Design review of the part built by this model. Coordinates are the model's own, in mm. A direction names the side the tool comes from. Coordinates: 2 decimals unless noted, no trailing zeros. Loops run counter-clockwise (first coordinate to the right, second up) from the corner with the lowest first, then second, coordinate; pieces in that order, holes last. Notation, with made-up numbers: (8, 44) - (52, 44) arc R4 cw to (52, 51) - close; hole circle Ø6 at (35, 86). An arc over 180 degrees is marked (long way). Use one line per item in the form item = value. Start each with the question number.
(1) Add section D-D (z = 11). State the section outline as (x, y) points.
(2) The part is to be moulded in two halves that separate along Y. For faces 5 (the face through (55, -3, 5)), 6 (the face through (-1, 12.5, 5)), 7 (the face through (0, 9, 10)), say which applies: pulls with the +Y half, pulls with the -Y half, needs draft (parallel to the pull), parting line crosses it, or undercut.
(3) Tool access review of faces 1 (the face through (-1, -10.5, 11)), 2 (the face through (57, -0.2, 4.6)), 3 (the face through (1, 0, 4)), 4 (the face through (0, 1, 7)): name each direction out of +Z, -Z, +X, -X, +Y, -Y from which nothing blocks a thin tool from reaching the whole face with its end or side.
(4) Add section B-B (y = 2). State the section outline as (x, z) points, plus the area to 3 significant figures.
(5) Clearance check with flat-ended pins moving along their axes: pin 1 Ø0.9 at (x, y) = (-55.5, -2.5) entering from +Z; pin 2 Ø0.6 at (x, z) = (2, 10.5) entering from +Y; pin 3 Ø1.5 at (x, y) = (6.5, -9.5) entering from +Z. State where each tip first meets the part, or that it passes through.
(6) For L1, parallel to X at y = 9, z = 9.25; L2, parallel to Y at x = -51, z = 2.75; L3, parallel to Z at x = 51.5, y = 11.25, list the stretches that pass through material, from the lowest coordinate up.
(7) Add section C-C (x = -28). State the section outline as (y, z) points.
(8) Add section A-A (z = 6.75). State the section outline as (x, y) points.
```python
from build123d import *

# Parameters (mm, degrees)
SKETCH1_W           = 114
SKETCH1_H           = 25
SKETCH1_W_2         = 108
SKETCH1_H_2         = 19
SKETCH1_W_3         = 2
BOSS_EXTRUDE1_DEPTH = 10
SKETCH2_W           = 114
SKETCH2_H           = 2
BOSS_EXTRUDE2_DEPTH = 2
SKETCH3_W           = 5
SKETCH3_H           = 8
CUT_EXTRUDE1_DEPTH  = 116.309366489


with BuildPart() as part:
    # Sketch1 → Boss-Extrude1 (new body)
    # profile 1 of 2: a face of its own
    with BuildSketch(Plane.XY):
        Rectangle(SKETCH1_W, SKETCH1_H)
        Rectangle(SKETCH1_W_2, SKETCH1_H_2, mode=Mode.SUBTRACT)
    # profile 2 of 2: a face of its own
    with BuildSketch(Plane.XY):
        Rectangle(SKETCH1_W_3, SKETCH1_H_2)
    extrude(amount=BOSS_EXTRUDE1_DEPTH)

    # Sketch2 → Boss-Extrude2 (add)
    with BuildSketch(Plane.XY.offset(10)):
        with Locations((0, -11.5)):
            Rectangle(SKETCH2_W, SKETCH2_H)
    extrude(amount=BOSS_EXTRUDE2_DEPTH)

    # Sketch3 → Cut-Extrude1 (cut, through all)
    with BuildSketch(Plane.ZY.offset(57)):
        with Locations((7.5, -3)):
            Rectangle(SKETCH3_W, SKETCH3_H)
    extrude(amount=-CUT_EXTRUDE1_DEPTH, mode=Mode.SUBTRACT)


solid = part.part
```
Computed values:
q1.outline = (-57, -12.5) - (57, -12.5) - (57, -10.5) - (-57, -10.5) - close
q2.face_5 = undercut
q2.face_6 = pulls with the +Y half
q2.face_7 = needs draft
q3.face_1 = +Z, +X, -X, +Y
q3.face_2 = +Z, -Z, +X, +Y, -Y
q3.face_3 = +Z, -Z
q3.face_4 = +Z, +X, -X
q4.outline = (-57, 0) - (-54, 0) - (-54, 10) - (-57, 10) - close; (-1, 0) - (1, 0) - (1, 10) - (-1, 10) - close; (54, 0) - (57, 0) - (57, 10) - (54, 10) - close
q4.area = 80.0 mm^2
q5.pin_1 = 5
q5.pin_2 = -10.5
q5.pin_3 = 10
q6.L1 = -57 to -54, -1 to 1, 54 to 57
q6.L2 = -12.5 to -9.5, 9.5 to 12.5
q6.L3 = 0 to 10
q7.outline = (-12.5, 0) - (-9.5, 0) - (-9.5, 10) - (-10.5, 10) - (-10.5, 12) - (-12.5, 12) - close; (9.5, 0) - (12.5, 0) - (12.5, 10) - (9.5, 10) - close
q8.outline = (-57, -12.5) - (57, -12.5) - (57, -7) - (54, -7) - (54, -9.5) - (1, -9.5) - (1, -7) - (-1, -7) - (-1, -9.5) - (-54, -9.5) - (-54, -7) - (-57, -7) - close; (-57, 1) - (-54, 1) - (-54, 9.5) - (-1, 9.5) - (-1, 1) - (1, 1) - (1, 9.5) - (54, 9.5) - (54, 1) - (57, 1) - (57, 12.5) - (-57, 12.5) - close
